Autodesk Inventor part; units mm, degrees
ref_plane "YZ Plane" through (0, 0, 0) normal (1, 0, 0) x (0, 1, 0)
ref_plane "XZ Plane" through (0, 0, 0) normal (0, 1, 0) x (-1, 0, 0)
ref_plane "XY Plane" through (0, 0, 0) normal (0, 0, 1) x (1, 0, 0)
ref_plane "Work Plane1" through (0, 69.5363, 0) normal (0, 0, 1) x (1, 0, 0)
sketch "Sketch1" plane through (0, 69.5363, 0) normal (0, 0, 1) x (1, 0, 0)
  line L0 (9.2773, 16.5681) -> (-0.7227, 16.5681)
  line L1 (0, -69.5363) -> (0, -2)
  line L2 (-20, 0) -> (-20, -2)
  line L3 (0, -2) -> (-20, -2)
  line L4 (-20, -2) -> (-20, 12)
  line L5 (-20, 12) -> (0, 12)
  line L6 (0, 12) -> (0, -2)
  dimension "d17" = 14
  dimension "d18" = 20
extrude "Extrusion1" add sketch "Sketch1" along normal blind -3.1173
sketch "Sketch2" plane through (0, 69.5363, -3.1173) normal (0, 0, -1) x (1, 0, 0)
  line L0 (0, 2) -> (-20, -12)
  line L1 (-20, 2) -> (0, -12)
  circle A0 centre (-10, -5) radius 1.5
  point P0 (0, 69.5363)
  point P1 (-10, 4)
  dimension "d22" = 3
extrude "Extrusion2" cut sketch "Sketch2" against normal up to surface (3.1173 mm away)
sketch "Sketch3" plane through (0, 69.5363, -3.1173) normal (0, 0, -1) x (1, 0, 0)
  line L0 (0, -12) -> (0, 2)
  line L1 (-20, 2) -> (-20, -12)
  line L2 (-20, 2) -> (0, -12) construction
  line L3 (-20, -12) -> (0, 2) construction
  line L4 (-20, -12) -> (-20, -14.5)
  line L5 (-20, -14.5) -> (-17.5, -14.5)
  line L6 (0, 2) -> (0, 4.5)
  line L7 (0, 4.5) -> (-2.5, 4.5)
  line L8 (-20, -12) -> (0, -12)
  line L9 (-14, 22) -> (-6, 22)
  line L10 (-6, 22) -> (-6, -12)
  line L11 (-6, -12) -> (-14, -12)
  line L12 (-14, -12) -> (-14, 22)
  line L13 (-14, 22) -> (-6, -12) construction
  line L14 (-6, 22) -> (-14, -12) construction
  line L15 (-20, 2) -> (0, 2)
  line L16 (0, 2) -> (0, -12)
  line L17 (0, -12) -> (-20, -12)
  line L18 (-20, -12) -> (-20, 2)
  point P0 (0, 69.5363)
  point P1 (-10, 5)
  dimension "d7" = 2.5
  dimension "d8" = 2.5
  dimension "d9" = 2.5
  dimension "d10" = 2.5
  dimension "d28" = 8
extrude "Extrusion4" cut sketch "Sketch3" against normal up to surface (3.1173 mm away) contours L8 L10 L15 L0 | L8 L1 L15 L12
sketch "Sketch4" plane through (-14, 67.5363, 0) normal (0, -1, 0) x (-1, 0, 0)
  line L0 (0, 0) -> (-8, 0)
  line L1 (-8, 0) -> (-8, 5)
  line L2 (-8, 5) -> (0, 5)
  line L3 (0, 5) -> (0, 0)
  point P0 (-14, 0)
  dimension "d34" = 5
extrude "Extrusion5" add sketch "Sketch4" along normal blind 2
sketch "Sketch5" plane through (-14, 81.5363, 0) normal (0, 1, 0) x (-1, 0, 0)
  line L0 (0, 0) -> (0, -5)
  line L1 (-8, 0) -> (0, 0)
  line L2 (0, 0) -> (0, -5)
  line L3 (0, -5) -> (-8, -5)
  line L4 (-8, -5) -> (-8, 0)
  dimension "d35" = 5
extrude "Extrusion6" add sketch "Sketch5" along normal blind 2
properties part number "pulley_housing_top"
For this review, take the finished solid that the model builds, in its own axes (mm). A direction names the side the tool comes from. Round coordinates to 2 decimals unless told otherwise and drop trailing zeros. Write each loop counter-clockwise with the first axis right and the second up, starting at its lowest first coordinate (ties: lowest second). Pieces come first, ordered by that corner, then holes. Notation, with made-up numbers: (65.5, 78) - (110.5, 78) arc R11 ccw to (110.5, 84) - close; hole circle Ø8 at (59, 82). An arc over 180 degrees is marked (long way). Use a Markdown table: item, result.
Q1. Wall thickness on line 1 along Y through (x, z) = (-10.5, -4.2); line 2 along Z through (x, y) = (-10.75, 79.25); line 3 along Y through (x, z) = (-9, -2.3): over which ranges is each line inside the solid? List them lowest first.
Derived:
| item | result |
|---|---|
| line 1 | y = 65.54 to 67.54, 81.54 to 83.54 |
| line 2 | z = -3.12 to 0 |
| line 3 | y = 65.54 to 73.42, 75.65 to 83.54 |
Q2. We need section B-B (z = -3.4). Give the boundary of the cut face in (x, y), plus the area to 3 significant figures.
Derived:
| item | result |
|---|---|
| outline | (-14, 65.54) - (-6, 65.54) - (-6, 67.54) - (-14, 67.54) - close; (-14, 81.54) - (-6, 81.54) - (-6, 83.54) - (-14, 83.54) - close |
| area | 32.0 mm2 |
Q3. The part is to be moulded in two halves that separate along Y. For faces 3 (the flat face through (-10, 83.536, -2)), 4 (the flat face through (-10, 65.536, -3)), 5 (the cylindrical face through (-11.19, 75.45, -1.58)), 6 (the flat face through (-14, 74, -2)), say which applies: pulls with the +Y half, pulls with the -Y half, needs draft (parallel to the pull), parting line crosses it, or undercut.
Derived:
| item | result |
|---|---|
| face 3 | pulls with the +Y half |
| face 4 | pulls with the -Y half |
| face 5 | undercut |
| face 6 | needs draft |
Q4. We need section C-C (y = 74). Give the boundary of the cut face in (x, z).
Derived:
| item | result |
|---|---|
| outline | (-14, -3.12) - (-11.4, -3.12) - (-11.4, 0) - (-14, 0) - close; (-8.6, -3.12) - (-6, -3.12) - (-6, 0) - (-8.6, 0) - close |
Q5. Clearance check with a flat-ended pin moving along its axis: pin 1 (4 mm diameter, centred on x = -12, y = 72.5, fed in from -Z). State where the tip first meets the part, or that it passes through.
Derived:
| item | result |
|---|---|
| pin 1 | stops at z = -3.12 |
Q6. We need section D-D (x = -12.25). Give the boundary of the cut face in (y, z).
Derived:
| item | result |
|---|---|
| outline | (65.54, -5) - (67.54, -5) - (67.54, -3.12) - (81.54, -3.12) - (81.54, -5) - (83.54, -5) - (83.54, 0) - (65.54, 0) - close |
Q7. Machinability: for faces 1 (the flat face through (-10, 67, -5)), 2 (the flat face through (-10, 81.536, -4)), which of the approach directions +Z, -Z, +X, -X, +Y, -Y give a long, thin tool a straight path to every point of the face, cutting with its end or side? Answer none if there is none.
Derived:
| item | result |
|---|---|
| face 1 | -Z, +X, -X, +Y, -Y |
| face 2 | -Z, +X, -X |
Q8. We need section A-A (x = -10). Give the boundary of the cut face in (y, z).
Derived:
| item | result |
|---|---|
| outline | (65.54, -5) - (67.54, -5) - (67.54, -3.12) - (73.04, -3.12) - (73.04, 0) - (65.54, 0) - close; (76.04, -3.12) - (81.54, -3.12) - (81.54, -5) - (83.54, -5) - (83.54, 0) - (76.04, 0) - close |
